Model file for the job. Use its own axes, mm. Face numbers are marked on the shaded views. A direction names the side the tool comes from. Give positions to 0.01 mm unless a question says otherwise; leave off trailing zeros. Loops run counter-clockwise (first coordinate to the right, second up) from the corner with the lowest first, then second, coordinate; pieces in that order, holes last. Notation, with made-up numbers: (-2.75, 89.25) - (47.25, 89.25) arc R21 ccw to (47.25, 120.25) - close; hole circle Ø5 at (31, 62). An arc over 180 degrees is marked (long way). Use a Markdown table: item, result.
from build123d import *

# Parameters (mm, degrees)
SKETCH1_R           = 12.5
SKETCH1_R_2         = 5.5
SKETCH1_R_3         = 1.75
BOSS_EXTRUDE1_DEPTH = 10
SKETCH3_R           = 2.6
BOSS_EXTRUDE2_DEPTH = 10
BOSS_EXTRUDE3_DEPTH = 20
SKETCH5_R           = 2.6
CUT_EXTRUDE1_DEPTH  = 42.122043967
FILLET3_R           = 3
FILLET4_R           = 3
RIB1_REACH          = 61.183
SKETCH6_WALL_W      = 132.856077754
SKETCH6_WALL_H      = 2
FILLET6_R           = 2
RIB2_START          = -2
RIB2_DEPTH          = 2
FILLET7_R           = 2
SKETCH8_R           = 5
CUT_EXTRUDE2_DEPTH  = 5


# Read off the part's stored shape, not the designer's step: Rib2
with BuildPart() as part:
    # Sketch1 → Boss-Extrude1 (new body)
    with BuildSketch(Plane(origin=(0, 0, 0), x_dir=(1, 0, 0), z_dir=(0, 1, 0))):
        with Locations(Location((0, 0, 0), (0, 0, 270))):
            Circle(SKETCH1_R)
        with Locations(Location((0, 0, 0), (0, 0, 270))):
            Circle(SKETCH1_R_2, mode=Mode.SUBTRACT)
        with Locations(Location((0, 8, 0), (0, 0, 270))):
            Circle(SKETCH1_R_3, mode=Mode.SUBTRACT)
        with Locations(Location((8, 0, 0), (0, 0, 270))):
            Circle(SKETCH1_R_3, mode=Mode.SUBTRACT)
        with Locations(Location((0, -8, 0), (0, 0, 270))):
            Circle(SKETCH1_R_3, mode=Mode.SUBTRACT)
        with Locations(Location((-8, 0, 0), (0, 0, 270))):
            Circle(SKETCH1_R_3, mode=Mode.SUBTRACT)
    extrude(amount=BOSS_EXTRUDE1_DEPTH)

    # Sketch3 → Boss-Extrude2 (add)
    with BuildSketch(Plane(origin=(0, 0, 0), x_dir=(1, 0, 0), z_dir=(0, 1, 0))):
        with BuildLine():
            Line((-12.5, 0), (-20, 22.35))
            Line((-20, 22.35), (-20, 42.35))
            Line((-20, 42.35), (20, 42.35))
            Line((20, 42.35), (20, 22.35))
            Line((20, 22.35), (12.5, 0))
            ThreePointArc((12.5, 0), (0, 12.5), (-12.5, 0))
        make_face()
        with Locations(Location((-10, 32.35, 0), (0, 0, 270))):
            Circle(SKETCH3_R, mode=Mode.SUBTRACT)
        with Locations(Location((10, 32.35, 0), (0, 0, 270))):
            Circle(SKETCH3_R, mode=Mode.SUBTRACT)
    extrude(amount=BOSS_EXTRUDE2_DEPTH)

    # Sketch4 → Boss-Extrude3 (add)
    with BuildSketch(Plane(origin=(0, 0, 0), x_dir=(1, 0, 0), z_dir=(0, 1, 0))):
        Polygon((20, 22.35), (-20, 22.35), (-18.322147651, 17.35), (18.322147651, 17.35), align=None)
    extrude(amount=-BOSS_EXTRUDE3_DEPTH)

    # Sketch5 → Cut-Extrude1 (cut, through all)
    with BuildSketch(Plane.XY.offset(-17.35)):
        with Locations((-10.822147651, -10)):
            Circle(SKETCH5_R)
        with Locations((10.822147651, -10)):
            Circle(SKETCH5_R)
    extrude(amount=-CUT_EXTRUDE1_DEPTH, mode=Mode.SUBTRACT)

    # Fillet3
    fillet3_edges = [part.edges().sort_by_distance(p)[0] for p in [
        (19.161073826, -20, -19.85),
        (-19.161073826, -20, -19.85),
    ]]
    fillet(fillet3_edges, radius=FILLET3_R)

    # Fillet4
    fillet4_edges = [part.edges().sort_by_distance(p)[0] for p in [
        (20, 5, -42.35),
        (-20, 5, -42.35),
    ]]
    fillet(fillet4_edges, radius=FILLET4_R)

    # Sketch6 wall → Rib1 (add, up to next)
    with BuildSketch(Plane(origin=(-16.866610739, -4.25, -13.0125), x_dir=(0.233087398642, 0.680588335288, 0.694600448074), z_dir=(-0.216519610858, 0.732666034336, -0.645228440356)), mode=Mode.PRIVATE) as rib1_sk1:
        with Locations((0, 1)):
            Rectangle(SKETCH6_WALL_W, SKETCH6_WALL_H)
    rib1_tool1 = extrude(rib1_sk1.sketch, amount=RIB1_REACH, mode=Mode.PRIVATE) - part.part
    add(rib1_tool1.solids().sort_by_distance((-16.866610739, -4.25, -13.0125))[0])

    # Fillet6
    fillet6_edges = [part.edges().sort_by_distance(p)[0] for p in [
        (-14.463028721, 0, -8.993135942),
        (-17.267345518, -8.188281786, -17.35),
    ]]
    fillet(fillet6_edges, radius=FILLET6_R)

    # Rib2 outline → Rib2 (add)
    with BuildSketch(Plane(origin=(11.234869034, 0, 3.77009028), x_dir=(0.31813594155425295, 0, -0.9480451058316736), z_dir=(0.9480451058316735, 0, 0.3181359415542529)).offset(RIB2_START)):
        Polygon((13.127107775, 0), (22.27751628, -8.5), (22.815775604, -9), (23, -9), (23, 1), (13, 1), (13, 0.11807299), align=None)
    extrude(amount=RIB2_DEPTH)

    # Fillet7
    fillet7_edges = [part.edges().sort_by_distance(p)[0] for p in [
        (17.267345517, -8.188281787, -17.35),
        (14.46302872, 0, -8.993135942),
    ]]
    fillet(fillet7_edges, radius=FILLET7_R)

    # Sketch8 → Cut-Extrude2 (cut)
    with BuildSketch(Plane(origin=(0, 10, 0), x_dir=(1, 0, 0), z_dir=(0, 1, 0))):
        with Locations(Location((-10, 32.35, 0), (0, 0, 270))):
            Circle(SKETCH8_R)
        with Locations(Location((10, 32.35, 0), (0, 0, 270))):
            Circle(SKETCH8_R)
    extrude(amount=-CUT_EXTRUDE2_DEPTH, mode=Mode.SUBTRACT)


solid = part.part
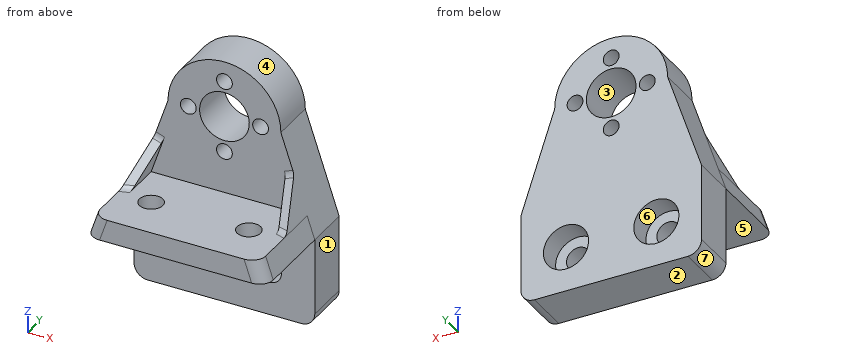
(1) Slice it at D-D, the plane x = 1. Write the cut outline in (y, z).
Computed:
| item | result |
|---|---|
| outline | (-20, -22.35) - (0, -22.35) - (0, -42.35) - (10, -42.35) - (10, -9.44) - (0, -9.44) - (0, -17.35) - (-20, -17.35) - close; (0, -6.56) - (10, -6.56) - (10, -5.41) - (0, -5.41) - close; (0, 5.41) - (10, 5.41) - (10, 6.56) - (0, 6.56) - close; (0, 9.44) - (10, 9.44) - (10, 12.46) - (0, 12.46) - close |
(2) Mould opens along Z. For the marked faces 1, 2, 3 and 4 say: pulls with the +Z half, pulls with the -Z half, needs draft (parallel to the pull), parting line crosses it, or undercut.
Computed:
| item | result |
|---|---|
| face 1 | needs draft |
| face 2 | pulls with the -Z half |
| face 3 | undercut |
| face 4 | pulls with the +Z half |
(3) Slice it at C-C, the plane y = -14.75. Write the cut outline in (x, z).
Computed:
| item | result |
|---|---|
| outline | (-20, -22.35) - (20, -22.35) - (18.32, -17.35) - (-18.32, -17.35) - close |
(4) Drill centre lines: probe 1 along X at (y, z) = (3.5, 0); probe 2 along X at (y, z) = (2.75, -32.35); probe 3 along Y at (x, z) = (-3, -7). Where is each one in solid material? Low to high. Write a range as [from, to].
Computed:
| item | result |
|---|---|
| probe 1 | [-12.5, -9.75], [-6.25, -5.5], [5.5, 6.25], [9.75, 12.5] |
| probe 2 | [-20, -12.6], [-7.4, 7.4], [12.6, 20] |
| probe 3 | [0, 10] |
(5) 3-axis set-ups, long thin cutter, end or side, ignore diameter. For the marked faces 5, 6 and 7: which of +Z, -Z, +X, -X, +Y, -Y reach the whole face in a straight line?
Computed:
| item | result |
|---|---|
| face 5 | -Z, +X, -X, -Y |
| face 6 | +Y |
| face 7 | -Z, -X, +Y, -Y |
(6) Slice it at A-A, the plane z = -33. Write the cut outline in (x, y), plus the area to 4 significant figures.
Computed:
| item | result |
|---|---|
| outline | (-20, 0) - (-12.52, 0) - (-12.52, 5) - (-14.96, 5) - (-14.96, 10) - (-20, 10) - close; (-7.48, 0) - (7.48, 0) - (7.48, 5) - (5.04, 5) - (5.04, 10) - (-5.04, 10) - (-5.04, 5) - (-7.48, 5) - close; (12.52, 0) - (20, 0) - (20, 10) - (14.96, 10) - (14.96, 5) - (12.52, 5) - close |
| area | 250.5 mm² |
(7) Slice it at B-B, the plane x = -3. Write the cut outline in (y, z), plus the area to 3 significant figures.
Computed:
| item | result |
|---|---|
| outline | (-20, -22.35) - (0, -22.35) - (0, -42.35) - (10, -42.35) - (10, -4.61) - (0, -4.61) - (0, -17.35) - (-20, -17.35) - close; (0, 4.61) - (10, 4.61) - (10, 12.13) - (0, 12.13) - close |
| area | 553 mm² |
(8) Pin check, flat tips, straight feed: P1, Ø4.5, axis at x = -8, z = 0, coming from the -Y side; P2, Ø3, axis at x = -8, y = -15.5, coming from the -Z side; P3, Ø3, axis at x = -8.5, z = -33, coming from the +Y side. Stop position of each tip, or through.
Computed:
| item | result |
|---|---|
| P1 | y = 0 |
| P2 | z = -22.35 |
| P3 | y = 5 |
